Verification items for the finished model (mm, model axes). Face numbers are marked on the shaded views. A direction names the side the tool comes from. Coordinates: 2 decimals unless noted, no trailing zeros. Loops run counter-clockwise (first coordinate to the right, second up) from the corner with the lowest first, then second, coordinate; pieces in that order, holes last. Notation, with made-up numbers: (34.25, 87.25) -> (52.25, 87.25) arc R26 ccw to (52.25, 110.25) -> close; hole circle Ø8 at (78, 39). An arc over 180 degrees is marked (long way). Write item = value, one per line.
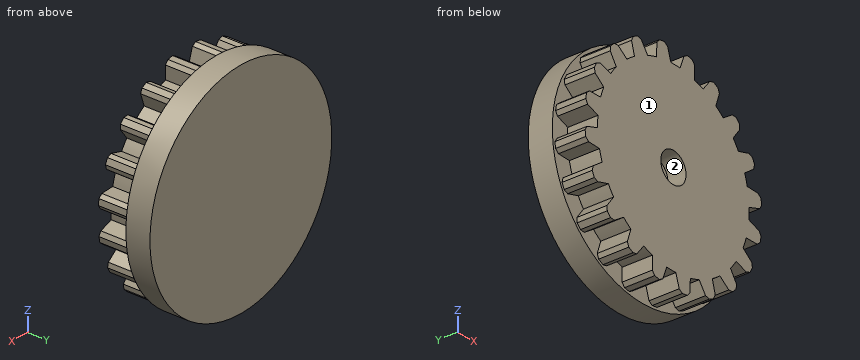
```python
from build123d import *

# Parameters (mm, degrees)
BOSS_EXTRUDE2_DEPTH = 127
SKETCH3_R           = 457.2
BOSS_EXTRUDE3_DEPTH = 101.6
SKETCH4_R           = 63.5
CUT_EXTRUDE1_DEPTH  = 76.2


with BuildPart() as part:
    # Sketch1 → Boss-Extrude2 (new body)
    with BuildSketch(Plane(origin=(0, 0, 0), x_dir=(1, 0, 0), z_dir=(0, 1, 0))):
        with BuildLine():
            Line((-358.285919954, 129.584719634), (-403.302421761, 161.579989966))
            Line((-403.302421761, 161.579989966), (-408.206038182, 180.409487441))
            Line((-408.206038182, 180.409487441), (-397.783371142, 202.356473607))
            Line((-397.783371142, 202.356473607), (-380.091440099, 210.455301))
            Line((-380.091440099, 210.455301), (-326.846738593, 195.786131968))
            ThreePointArc((-326.846738593, 195.786131968), (-314.356463225, 215.269630995), (-300.706278291, 233.958830131))
            Line((-300.706278291, 233.958830131), (-333.632433402, 278.299004557))
            Line((-333.632433402, 278.299004557), (-332.477415039, 297.722221637))
            Line((-332.477415039, 297.722221637), (-315.782877932, 315.374264601))
            Line((-315.782877932, 315.374264601), (-296.454176329, 317.609599812))
            Line((-296.454176329, 317.609599812), (-250.348478528, 287.20487339))
            ThreePointArc((-250.348478528, 287.20487339), (-232.44878844, 301.875074746), (-213.691410965, 315.431420248))
            Line((-213.691410965, 315.431420248), (-231.304177909, 367.776173558))
            Line((-231.304177909, 367.776173558), (-224.203586005, 385.891830426))
            Line((-224.203586005, 385.891830426), (-202.871356441, 397.521025234))
            Line((-202.871356441, 397.521025234), (-183.797912262, 393.674058078))
            Line((-183.797912262, 393.674058078), (-149.344365104, 350.51000073))
            ThreePointArc((-149.344365104, 350.51000073), (-127.787406676, 358.930882894), (-105.758939458, 366.027385211))
            Line((-105.758939458, 366.027385211), (-106.334257891, 421.252848245))
            Line((-106.334257891, 421.252848245), (-93.983147854, 436.287658187))
            Line((-93.983147854, 436.287658187), (-70.101373095, 440.755658225))
            Line((-70.101373095, 440.755658225), (-53.150227948, 431.202956651))
            Line((-53.150227948, 431.202956651), (-33.72138468, 379.504767052))
            ThreePointArc((-33.72138468, 379.504767052), (-10.617303199, 380.852035406), (12.525953909, 380.794039447))
            Line((12.525953909, 380.794039447), (29.044400164, 433.494359103))
            Line((29.044400164, 433.494359103), (45.437015627, 443.97661017))
            Line((45.437015627, 443.97661017), (69.530621076, 440.846056464))
            Line((69.530621076, 440.846056464), (82.700170997, 426.522705459))
            Line((82.700170997, 426.522705459), (85.202479827, 371.35096261))
            ThreePointArc((85.202479827, 371.35096261), (107.59209589, 365.49273714), (129.584719634, 358.285919954))
            Line((129.584719634, 358.285919954), (161.579989966, 403.302421761))
            Line((161.579989966, 403.302421761), (180.409487441, 408.206038182))
            Line((180.409487441, 408.206038182), (202.356473607, 397.783371142))
            Line((202.356473607, 397.783371142), (210.455301, 380.091440099))
            Line((210.455301, 380.091440099), (195.786131968, 326.846738593))
            ThreePointArc((195.786131968, 326.846738593), (215.269630995, 314.356463225), (233.958830131, 300.706278291))
            Line((233.958830131, 300.706278291), (278.299004557, 333.632433402))
            Line((278.299004557, 333.632433402), (297.722221637, 332.477415039))
            Line((297.722221637, 332.477415039), (315.374264601, 315.782877932))
            Line((315.374264601, 315.782877932), (317.609599812, 296.454176329))
            Line((317.609599812, 296.454176329), (287.20487339, 250.348478528))
            ThreePointArc((287.20487339, 250.348478528), (301.875074746, 232.44878844), (315.431420248, 213.691410965))
            Line((315.431420248, 213.691410965), (367.776173558, 231.304177909))
            Line((367.776173558, 231.304177909), (385.891830426, 224.203586005))
            Line((385.891830426, 224.203586005), (397.521025234, 202.871356441))
            Line((397.521025234, 202.871356441), (393.674058078, 183.797912262))
            Line((393.674058078, 183.797912262), (350.51000073, 149.344365104))
            ThreePointArc((350.51000073, 149.344365104), (358.930882894, 127.787406676), (366.027385211, 105.758939458))
            Line((366.027385211, 105.758939458), (421.252848245, 106.334257891))
            Line((421.252848245, 106.334257891), (436.287658187, 93.983147854))
            Line((436.287658187, 93.983147854), (440.755658225, 70.101373095))
            Line((440.755658225, 70.101373095), (431.202956651, 53.150227948))
            Line((431.202956651, 53.150227948), (379.504767052, 33.72138468))
            ThreePointArc((379.504767052, 33.72138468), (380.852035406, 10.617303199), (380.794039447, -12.525953909))
            Line((380.794039447, -12.525953909), (433.494359103, -29.044400164))
            Line((433.494359103, -29.044400164), (443.97661017, -45.437015627))
            Line((443.97661017, -45.437015627), (440.846056464, -69.530621076))
            Line((440.846056464, -69.530621076), (426.522705459, -82.700170997))
            Line((426.522705459, -82.700170997), (371.35096261, -85.202479827))
            ThreePointArc((371.35096261, -85.202479827), (365.49273714, -107.59209589), (358.285919954, -129.584719634))
            Line((358.285919954, -129.584719634), (403.302421761, -161.579989966))
            Line((403.302421761, -161.579989966), (408.206038182, -180.409487441))
            Line((408.206038182, -180.409487441), (397.783371142, -202.356473607))
            Line((397.783371142, -202.356473607), (380.091440099, -210.455301))
            Line((380.091440099, -210.455301), (326.846738593, -195.786131968))
            ThreePointArc((326.846738593, -195.786131968), (314.356463225, -215.269630995), (300.706278291, -233.958830131))
            Line((300.706278291, -233.958830131), (333.632433402, -278.299004557))
            Line((333.632433402, -278.299004557), (332.477415039, -297.722221637))
            Line((332.477415039, -297.722221637), (315.782877932, -315.374264601))
            Line((315.782877932, -315.374264601), (296.454176329, -317.609599812))
            Line((296.454176329, -317.609599812), (250.348478528, -287.20487339))
            ThreePointArc((250.348478528, -287.20487339), (232.44878844, -301.875074746), (213.691410965, -315.431420248))
            Line((213.691410965, -315.431420248), (231.304177909, -367.776173558))
            Line((231.304177909, -367.776173558), (224.203586005, -385.891830426))
            Line((224.203586005, -385.891830426), (202.871356441, -397.521025234))
            Line((202.871356441, -397.521025234), (183.797912262, -393.674058078))
            Line((183.797912262, -393.674058078), (149.344365104, -350.51000073))
            ThreePointArc((149.344365104, -350.51000073), (127.787406676, -358.930882894), (105.758939458, -366.027385211))
            Line((105.758939458, -366.027385211), (106.334257891, -421.252848245))
            Line((106.334257891, -421.252848245), (93.983147854, -436.287658187))
            Line((93.983147854, -436.287658187), (70.101373095, -440.755658225))
            Line((70.101373095, -440.755658225), (53.150227948, -431.202956651))
            Line((53.150227948, -431.202956651), (33.72138468, -379.504767052))
            ThreePointArc((33.72138468, -379.504767052), (10.617303199, -380.852035406), (-12.525953909, -380.794039447))
            Line((-12.525953909, -380.794039447), (-29.044400164, -433.494359103))
            Line((-29.044400164, -433.494359103), (-45.437015627, -443.97661017))
            Line((-45.437015627, -443.97661017), (-69.530621076, -440.846056464))
            Line((-69.530621076, -440.846056464), (-82.700170997, -426.522705459))
            Line((-82.700170997, -426.522705459), (-85.202479827, -371.35096261))
            ThreePointArc((-85.202479827, -371.35096261), (-107.59209589, -365.49273714), (-129.584719634, -358.285919954))
            Line((-129.584719634, -358.285919954), (-161.579989966, -403.302421761))
            Line((-161.579989966, -403.302421761), (-180.409487441, -408.206038182))
            Line((-180.409487441, -408.206038182), (-202.356473607, -397.783371142))
            Line((-202.356473607, -397.783371142), (-210.455301, -380.091440099))
            Line((-210.455301, -380.091440099), (-195.786131968, -326.846738593))
            ThreePointArc((-195.786131968, -326.846738593), (-215.269630995, -314.356463225), (-233.958830131, -300.706278291))
            Line((-233.958830131, -300.706278291), (-278.299004557, -333.632433402))
            Line((-278.299004557, -333.632433402), (-297.722221637, -332.477415039))
            Line((-297.722221637, -332.477415039), (-315.374264601, -315.782877932))
            Line((-315.374264601, -315.782877932), (-317.609599812, -296.454176329))
            Line((-317.609599812, -296.454176329), (-287.20487339, -250.348478528))
            ThreePointArc((-287.20487339, -250.348478528), (-301.875074746, -232.44878844), (-315.431420248, -213.691410965))
            Line((-315.431420248, -213.691410965), (-367.776173558, -231.304177909))
            Line((-367.776173558, -231.304177909), (-385.891830426, -224.203586005))
            Line((-385.891830426, -224.203586005), (-397.521025234, -202.871356441))
            Line((-397.521025234, -202.871356441), (-393.674058078, -183.797912262))
            Line((-393.674058078, -183.797912262), (-350.51000073, -149.344365104))
            ThreePointArc((-350.51000073, -149.344365104), (-358.930882894, -127.787406676), (-366.027385211, -105.758939458))
            Line((-366.027385211, -105.758939458), (-421.252848245, -106.334257891))
            Line((-421.252848245, -106.334257891), (-436.287658187, -93.983147854))
            Line((-436.287658187, -93.983147854), (-440.755658225, -70.101373095))
            Line((-440.755658225, -70.101373095), (-431.202956651, -53.150227948))
            Line((-431.202956651, -53.150227948), (-379.504767052, -33.72138468))
            ThreePointArc((-379.504767052, -33.72138468), (-380.852035406, -10.617303199), (-380.794039447, 12.525953909))
            Line((-380.794039447, 12.525953909), (-433.494359103, 29.044400164))
            Line((-433.494359103, 29.044400164), (-443.97661017, 45.437015627))
            Line((-443.97661017, 45.437015627), (-440.846056464, 69.530621076))
            Line((-440.846056464, 69.530621076), (-426.522705459, 82.700170997))
            Line((-426.522705459, 82.700170997), (-371.35096261, 85.202479827))
            ThreePointArc((-371.35096261, 85.202479827), (-365.49273714, 107.59209589), (-358.285919954, 129.584719634))
        make_face()
    extrude(amount=BOSS_EXTRUDE2_DEPTH)

    # Sketch3 → Boss-Extrude3 (add)
    with BuildSketch(Plane(origin=(0, 127, 0), x_dir=(1, 0, 0), z_dir=(0, 1, 0))):
        with Locations(Location((0, 0, 0), (0, 0, 270))):
            Circle(SKETCH3_R)
    extrude(amount=BOSS_EXTRUDE3_DEPTH)

    # Sketch4 → Cut-Extrude1 (cut)
    with BuildSketch(Plane(origin=(0, 0, 0), x_dir=(-1, 0, 0), z_dir=(0, -1, 0))):
        with Locations(Location((0, 0, 0), (0, 0, 90))):
            Circle(SKETCH4_R)
    extrude(amount=-CUT_EXTRUDE1_DEPTH, mode=Mode.SUBTRACT)


solid = part.part
```
1) Sectioned sample at B-B, the plane z = 0. Record the cut outline in (x, y), plus the area to 3 significant figures.
Ans:
outline = (-457.2, 127) -> (-381, 127) -> (-381, 0) -> (-63.5, 0) -> (-63.5, 76.2) -> (63.5, 76.2) -> (63.5, 0) -> (381, 0) -> (381, 127) -> (457.2, 127) -> (457.2, 228.6) -> (-457.2, 228.6) -> close
area = 180,000 mm2
2) Material ranges on line 1 (X direction, y = 54.5, z = 0); line 2 (Z direction, x = -410.5, y = 31.5); line 3 (Z direction, x = 136, y = 206), recorded low to high.
Ans:
line_1 = -381 to -63.5, 63.5 to 381
line_2 = -83.43 to -21.84, 45.37 to 106.22
line_3 = -436.5 to 436.5
3) Sectioned sample at A-A, the plane x = 0. Record the cut outline in (y, z), plus the area to 3 significant figures.
Ans:
outline = (0, -381) -> (127, -381) -> (127, -457.2) -> (228.6, -457.2) -> (228.6, 457.2) -> (127, 457.2) -> (127, 381) -> (0, 381) -> (0, 63.5) -> (76.2, 63.5) -> (76.2, -63.5) -> (0, -63.5) -> close
area = 180,000 mm2
4) Tool access check on the marked faces 1 and 2. Record the directions out of +Z, -Z, +X, -X, +Y, -Y that give a thin tool (end or side, any length) a straight path to the whole face; none if there is none.
Ans:
face_1 = +Z, -Z, +X, -X, -Y
face_2 = -Y
5) Depth check by flat-ended pin: pin 1 Ø12 at (x, y) = (-319, 93) entering from -Z; pin 2 Ø4 at (x, z) = (-353, -223.5) entering from -Y; pin 3 Ø5 at (x, y) = (26, 38.5) entering from +Z. Enter the tip coordinate at first touch or a pass-through.
Ans:
pin_1 = -315.7
pin_2 = 127
pin_3 = 380.27
